Autodesk Inventor part; units mm, degrees
ref_plane "YZ Plane" through (0, 0, 0) normal (1, 0, 0) x (0, 1, 0)
ref_plane "XZ Plane" through (0, 0, 0) normal (0, 1, 0) x (-1, 0, 0)
ref_plane "XY Plane" through (0, 0, 0) normal (0, 0, 1) x (1, 0, 0)
sketch "Sketch1" plane through (0, 0, 0) normal (0, 1, 0) x (-1, 0, 0)
  line L0 (-25, -100) -> (25, -100)
  line L1 (25, -100) -> (25, 100)
  line L2 (25, 100) -> (-25, 100)
  line L3 (-25, 100) -> (-25, -100)
  line L4 (-25, -100) -> (25, 100) construction
  line L5 (25, -100) -> (-25, 100) construction
  point P0 (0, 0)
  dimension "d0" = 50
  dimension "d1" = 200
extrude "Extrusion1" add sketch "Sketch1" along normal blind 5
sketch "Sketch2" plane through (0, 5, 0) normal (0, 1, 0) x (1, 0, 0)
  line L0 (22, 97) -> (-22, 97)
  line L1 (22, -97) -> (22, 97)
  line L2 (-25, -100) -> (25, -100)
  line L3 (25, -100) -> (25, 100)
  line L4 (19, 94) -> (-22, 94)
  line L5 (19, -94) -> (19, 94)
  line L6 (25, 100) -> (-25, 100)
  line L7 (-22, 97) -> (-22, 94)
  line L8 (-25, 100) -> (-25, -100)
  line L9 (22, -97) -> (-22, -97)
  line L10 (22, -97) -> (66, -97) construction
  line L11 (19, -94) -> (-22, -94)
  line L12 (19, -94) -> (60, -94) construction
  line L13 (-22, -94) -> (-22, -97)
  point P0 (0, 0)
  dimension "d5" = 3
  dimension "d6" = 3
  dimension "d10" = 3
  dimension "d11" = 3
  dimension "d12" = 3
  dimension "d33" = 3
  dimension "d34" = 3
  dimension "d35" = 3
extrude "Extrusion2" add sketch "Sketch2" along normal blind 25 contours L1 L9 L13 L11 L5 L4 L7 L0
fillet "Fillet1" radius 2 4 edges at (22, 17.5, 97) (22, 17.5, -97) (-22, 17.5, -97) (-22, 17.5, 97)
sketch "Sketch3" plane through (22, 5, 95) normal (1, 0, 0) x (0, 0, -1)
  line L0 (185, 22.5) -> (5, 22.5)
  line L1 (5, 22.5) -> (5, 2.5)
  line L2 (5, 2.5) -> (185, 2.5)
  line L3 (185, 2.5) -> (185, 22.5)
  line L4 (185, 22.5) -> (5, 2.5) construction
  line L5 (5, 22.5) -> (185, 2.5) construction
  line L6 (-5, -5) -> (-5, 0)
  line L7 (195, -5) -> (195, 0)
  line L8 (0, 0) -> (0, 25)
  point P0 (95, -5)
  point P1 (95, 12.5)
  point P2 (0, 12.5)
  dimension "d15" = 10
  dimension "d16" = 10
  dimension "d17" = 20
  dimension "d18" = 10
extrude "Extrusion3" add sketch "Sketch3" along normal blind 6
sketch "Sketch4" plane through (22, 7.5, -90) normal (0, 0, -1) x (-1, 0, 0)
  line L0 (0, 20) -> (0, 0)
  line L1 (0, 20) -> (-6, 20)
  line L2 (-6, 0) -> (-6, 20)
  line L3 (0, 0) -> (-6, 0)
  line L4 (-6, 7.5) -> (-3, 7.5)
  line L5 (-3, 7.5) -> (-3, 12.5)
  line L6 (-3, 12.5) -> (-6, 12.5)
  line L7 (-6, 12.5) -> (-6, 7.5)
  line L8 (0, 5) -> (-3, 5)
  line L9 (-3, 5) -> (-3, 15)
  line L10 (-3, 15) -> (0, 15)
  line L11 (0, 15) -> (0, 5)
  point P0 (22, -7.5)
  point P1 (0, 15)
  point P2 (-3, 12.5)
  point P3 (-6, 12.5)
  point P4 (-3, 7.5)
  dimension "d22" = 3
  dimension "d23" = 3
  dimension "d24" = 2.5
  dimension "d25" = 2.5
  dimension "d26" = 5
  dimension "d27" = 5
extrude "Extrusion4" cut sketch "Sketch4" against normal blind 170 contours L0 L8 L9 L5 L10 | L6 L5 L4 L2
fillet "Fillet2" radius 2 3 edges at (28, 17.5, 90) (28, 23.75, -90) (28, 11.25, -90)
properties part number "module_valve"
CAD build for the part. Positions are in the model's coordinates, mm. A direction names the side the tool comes from. Round coordinates to 2 decimals unless told otherwise and drop trailing zeros. Write each loop counter-clockwise with the first axis right and the second up, starting at its lowest first coordinate (ties: lowest second). Pieces come first, ordered by that corner, then holes. Notation, with made-up numbers: (-13, 45.5) -> (-6, 45.5) arc R17 cw to (-6, 63.5) -> close; hole circle Ø3 at (5, 18). An arc over 180 degrees is marked (long way). Answer as a JSON object with one key per item and string values.
(1) Band-saw the part on B-B, the plane x = 16. List the corners of the cut face in (y, z), then the cut area to 3 significant figures.
Reported:
{"outline": "(0, -100) -> (5, -100) -> (5, -97) -> (30, -97) -> (30, -94) -> (5, -94) -> (5, 94) -> (30, 94) -> (30, 97) -> (5, 97) -> (5, 100) -> (0, 100) -> close", "area": "1,150 mm^2"}
(2) Pin check, flat tips, straight feed: P1, Ø1, axis at y = 17.5, z = -55, coming from the -X side; P2, Ø4, axis at x = -17.5, z = -8, coming from the +Y side; P3, Ø0.8, axis at y = 16, z = 94.5, coming from the -X side. Stop position of each tip, or through.
Reported:
{"P1": "stops at x = 19", "P2": "stops at y = 5", "P3": "stops at x = -22"}
(3) Band-saw the part on D-D, the plane z = 85. List the corners of the cut face in (x, y).
Reported:
{"outline": "(-25, 0) -> (25, 0) -> (25, 5) -> (22, 5) -> (22, 7.5) -> (28, 7.5) -> (28, 27.5) -> (22, 27.5) -> (22, 30) -> (19, 30) -> (19, 5) -> (-25, 5) -> close"}
(4) Band-saw the part on A-A, the plane z = 17.5. List the corners of the cut face in (x, y), then the cut area to 3 significant figures.
Reported:
{"outline": "(-25, 0) -> (25, 0) -> (25, 5) -> (22, 5) -> (22, 7.5) -> (28, 7.5) -> (28, 15) -> (25, 15) -> (25, 12.5) -> (22, 12.5) -> (22, 22.5) -> (25, 22.5) -> (25, 20) -> (28, 20) -> (28, 27.5) -> (22, 27.5) -> (22, 30) -> (19, 30) -> (19, 5) -> (-25, 5) -> close", "area": "400 mm^2"}
(5) Which spindle directions (+Z, -Z, +X, -X, +Y, -Y) get a long thin tool onto all of the face, cutting with end or side? Do faces 4 (the face through (25, 27.5, -1)), 5 (the face through (24, 18, 90)), 6 (the face through (25, 7.5, 1)), 7 (the face through (24, 25, -90)). Say none if no direction does.
Reported:
{"face 4": "+Z, -Z, +X, +Y", "face 5": "+Z, +X, +Y", "face 6": "+Z, -Z, +X", "face 7": "-Z, +X, +Y"}
(6) Two-plate mould, pull along X, no slides. Class faces 1 (the face through (24, 18, 80)), 2 (the face through (19, 17, 1)), 3 (the face through (0, 2, 100)): +X half, -X half, draft (parallel to the pull), parting line (faces both ways), or undercut.
Reported:
{"face 1": "undercut", "face 2": "-X half", "face 3": "draft"}
(7) Probe probe 1 along Y at (x, z) = (22.5, -76.5); probe 2 along X at (y, z) = (21.5, -73); probe 3 along Z at (x, y) = (-2, 26). List the from-to ranges inside material, lowest first. Write a range as [from, to].
Reported:
{"probe 1": "y = [0, 5], [7.5, 12.5], [22.5, 27.5]", "probe 2": "x = [19, 22], [25, 28]", "probe 3": "z = [-97, -94], [94, 97]"}
(8) Band-saw the part on C-C, the plane y = 2.25. List the corners of the cut face in (x, z).
Reported:
{"outline": "(-25, -100) -> (25, -100) -> (25, 100) -> (-25, 100) -> close"}
